from build123d import *

# Parameters (mm, degrees)
SKETCH1_W                       = 89
SKETCH1_H                       = 44
BOSS_EXTRUDE1_DEPTH             = 30
SKETCH3_R                       = 14
CUT_EXTRUDE1_DEPTH              = 97.462427919
F_5_0MM_DOWEL_HOLE1_D           = 5
F_5_0MM_DOWEL_HOLE1_CSINK_D     = 5.05
F_5_0MM_DOWEL_HOLE1_CSINK_ANGLE = 90


with BuildPart() as part:
    # Sketch1 → Boss-Extrude1 (new, symmetric)
    with BuildSketch(Plane.XY):
        Rectangle(SKETCH1_W, SKETCH1_H)
    extrude(amount=BOSS_EXTRUDE1_DEPTH, both=True)

    # Sketch3 → Cut-Extrude1 (cut, through all)
    with BuildSketch(Plane.ZY.offset(44.5)):
        with Locations(Location((0, 0, 0), (0, 0, 270))):
            Circle(SKETCH3_R)
    extrude(amount=-CUT_EXTRUDE1_DEPTH, mode=Mode.SUBTRACT)

    # Ø5.0mm Dowel Hole1 (through all)
    with Locations(Plane(origin=(0, 22, 0), x_dir=(1, 0, 0), z_dir=(0, 1, 0))):
        with Locations((-35.759887734, 20.696035026)):
            CounterSinkHole(F_5_0MM_DOWEL_HOLE1_D / 2, F_5_0MM_DOWEL_HOLE1_CSINK_D / 2, counter_sink_angle=F_5_0MM_DOWEL_HOLE1_CSINK_ANGLE)


solid = part.part
Work out the finished part from the listing and answer in its coordinate system (mm). Give positions to 0.01 mm unless a question says otherwise; leave off trailing zeros. Write each loop counter-clockwise with the first axis right and the second up, starting at its lowest first coordinate (ties: lowest second). Pieces come first, ordered by that corner, then holes.
Q1. For a pull along Z with two mould halves and no side action, classify faces 1 (the face through (-1, 0, -30)), 2 (the face through (-0.62, 3.03, -13.67)), 3 (the face through (44.5, -5, 14)), 4 (the face through (-38.07, -0.32, -19.74)) as released by +Z, released by -Z, zero draft, split by the parting line, or undercut.
Answer:
face 1: released by -Z
face 2: undercut
face 3: zero draft
face 4: undercut
Q2. The part is cut by section D-D on y = 0. Give the vertices of the cut face in (x, z), and give its area (3 significant figures).
Answer:
outline: (-44.5, -30) - (44.5, -30) - (44.5, -14) - (-44.5, -14) - close; (-44.5, 14) - (44.5, 14) - (44.5, 30) - (-44.5, 30) - close; hole circle Ø5 at (-35.76, -20.7)
area: 2,830 mm2
Q3. The part is cut by section B-B on z = 0. Give the vertices of the cut face in (x, y), and give its area (3 significant figures).
Answer:
outline: (-44.5, -22) - (44.5, -22) - (44.5, -14) - (-44.5, -14) - close; (-44.5, 14) - (44.5, 14) - (44.5, 22) - (-44.5, 22) - close
area: 1,420 mm2
Q4. The part is cut by section C-C on x = -15. Give the vertices of the cut face in (y, z), and give its area (3 significant figures).
Answer:
outline: (-22, -30) - (22, -30) - (22, 30) - (-22, 30) - close; hole circle Ø28 at (0, 0)
area: 2,020 mm2
Q5. Given pin 1 (1 mm diameter, centred on y = -1, z = 13, fed in from +X), flat-ended and moving along its own axis, determine where the tip first touches the part or whether it passes through.
Answer:
pin 1: passes through
Q6. Straight lines are drawn through the part: L1, parallel to Y at x = 23, z = -0.5; L2, parallel to Z at x = -33.5, y = -11.5; L3, parallel to Z at x = 1.5, y = -9. For each, find the intervals that lie inside material, in ascending order.
Answer:
L1: y = -22 to -13.99, 13.99 to 22
L2: z = -30 to -21.77, -19.63 to -7.98, 7.98 to 30
L3: z = -30 to -10.72, 10.72 to 30
Q7. The part is cut by section A-A on y = 11. Give the vertices of the cut face in (x, z), and give its area (3 significant figures).
Answer:
outline: (-44.5, -30) - (44.5, -30) - (44.5, -8.66) - (-44.5, -8.66) - close; (-44.5, 8.66) - (44.5, 8.66) - (44.5, 30) - (-44.5, 30) - close; hole circle Ø5 at (-35.76, -20.7)
area: 3,780 mm2
